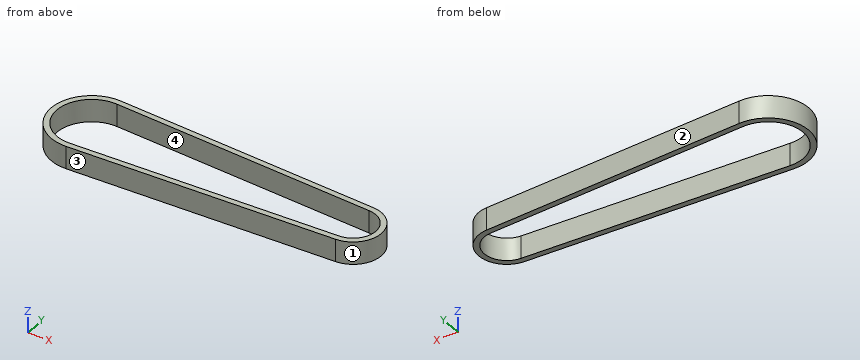
Autodesk Inventor part; units mm, degrees
ref_plane "YZ Plane" through (0, 0, 0) normal (1, 0, 0) x (0, 1, 0)
ref_plane "XZ Plane" through (0, 0, 0) normal (0, 1, 0) x (-1, 0, 0)
ref_plane "XY Plane" through (0, 0, 0) normal (0, 0, 1) x (1, 0, 0)
sketch "スケッチ1" plane through (0, 0, 0) normal (0, 0, 1) x (1, 0, 0)
  arc A0 (0.4385, 9.2897) -> (0.4384, -9.2897) centre (0, 0) ccw
  arc A1 (0.5091, 10.788) -> (0.5091, -10.788) centre (0, 0) ccw
  arc A2 (70.3536, -7.4917) -> (70.3536, 7.4917) centre (70, 0) ccw
  line L0 (0.5091, 10.788) -> (70.3536, 7.4917)
  line L1 (70.3536, -7.4917) -> (0.5091, -10.788)
  line L2 (70.1922, 5.9969) -> (0.4385, 9.2897)
  circle A3 centre (70, 0) radius 6
  line L3 (0.4384, -9.2897) -> (70.2829, -5.9933)
  point P0 (1.0111, -13.9634)
  point P1 (90.5417, -7.4804)
  point P2 (90.5417, 7.4804)
  point P3 (1.0111, 13.9634)
  point P4 (0.9028, 12.4674)
  dimension "d0" = 18.6
  dimension "d2" = 70
  dimension "d3" = 1.5
  dimension "d7" = 12
  dimension "d8" = 1.5
extrude "押し出し1" add sketch "スケッチ1" along normal blind 6
properties part number "Bed_Unit_Belt" material "ゴム"
Work out the finished part from the listing and answer in its coordinate system (mm). Face numbers are marked on the shaded views. Coordinates: 2 decimals unless noted, no trailing zeros. Write each loop counter-clockwise with the first axis right and the second up, starting at its lowest first coordinate (ties: lowest second). Pieces come first, ordered by that corner, then holes.
Q1. Determine the mould class of the marked faces 1, 2, 3 and 4 for opening direction Y: released by +Y, released by -Y, zero draft, split by the parting line, or undercut.
Q2. A cutting plane is placed at C-C, the plane z = 1.25. Give the vertices of the cut face in (x, y), then the cut area to 3 significant figures.
Q3. Each of these flat-tipped pins is pushed along its axis until it touches: pin 1 Ø1 at (y, z) = (-2.5, 1) entering from -X; pin 2 Ø2 at (y, z) = (3.5, 0.5) entering from -X. Where does it stop, or does it pass through?
Q4. Find the intervals of material crossed by line 1 (Y direction, x = 0, z = 2.9); line 2 (Y direction, x = 27, z = 2); line 3 (X direction, y = -2.5, z = 1.85), in increasing order.
Q5. A cutting plane is placed at A-A, the plane y = 0. Give the vertices of the cut face in (x, z).
Q6. A cutting plane is placed at B-B, the plane x = 27. Give the vertices of the cut face in (y, z).
Findings below:
1. face 1: split by the parting line
1. face 2: released by +Y
1. face 3: released by -Y
1. face 4: undercut
2. outline: (0.51, -10.79) - (70.35, -7.49) arc R7.5 ccw to (70.35, 7.49) - (0.51, 10.79) arc R10.8 ccw (long way) to start; hole (0.44, -9.29) - (70.28, -5.99) arc R6 ccw to (70.19, 6) - (0.44, 9.29) arc R9.3 ccw (long way) to start
2. area: 289 mm2
3. pin 1: stops at x = -10.61
3. pin 2: stops at x = -10.51
4. line 1: y = -10.8 to -9.3, 9.3 to 10.8
4. line 2: y = -9.54 to -8.04, 8.04 to 9.54
4. line 3: x = -10.51 to -8.96, 75.45 to 77.07
5. outline: (-10.8, 0) - (-9.3, 0) - (-9.3, 6) - (-10.8, 6) - close; (76, 0) - (77.5, 0) - (77.5, 6) - (76, 6) - close
6. outline: (-9.54, 0) - (-8.04, 0) - (-8.04, 6) - (-9.54, 6) - close; (8.04, 0) - (9.54, 0) - (9.54, 6) - (8.04, 6) - close
